Part model, mm, in its own coordinate system. Give positions to 0.01 mm unless a question says otherwise; leave off trailing zeros. Order: outer loops, then holes, each group sorted by start corner. A loop starts at its lowest first (then second) coordinate and runs counter-clockwise, first axis right, second up. Notation, with made-up numbers: (-24, 26) -> (5, 26) arc R12 ccw to (5, 36) -> close; hole circle Ø9 at (13, -31.5). An arc over 180 degrees is marked (long way). Write item = value, one per line. Start each with the question number.
Item 1: Drill centre lines: line 1 along Y through (x, z) = (-13.5, 0.5); line 2 along X through (y, z) = (5.5, -1.3); line 3 along Y through (x, z) = (-2, 0.4). Where is each one in solid material? Low to high.
Item 2: Pull direction X, two halves, no side cores. Call faces 1 (the face through (2, 0, -4)), 2 (the face through (14.219, -14.943, -1.535)), 3 (the face through (-21.083, 0, -2)), 4 (the face through (24.984, -0.901, -1.535)): +X half, -X half, draft (parallel to the pull), parting line (faces both ways), or undercut.
Item 3: Flat gauge pins, fed straight in: P1, Ø1.5, axis at x = 18.5, z = 0.5, coming from the +Y side; P2, Ø1, axis at x = 12.5, z = -2, coming from the -Y side. Where does each tip first touch, or does it go through?
Item 4: Band-saw the part on C-C on y = 21. Write the cut outline in (x, z).
Item 5: Band-saw the part on B-B on x = 20. Write the cut outline in (y, z).
Item 6: Band-saw the part on A-A on z = -2.45. Write the cut outline in (x, y), plus the area to 3 significant figures.
```python
from build123d import *

# Parameters (mm, degrees)
BOSS_EXTRU_1_DEPTH      = 1
BOSS_EXTRU_1_DEPTH_BACK = 4
ESQUISSE1_R             = 25
ESQUISSE1_R_2           = 1.7
ESQUISSE2_W             = 7.120092975
ESQUISSE2_H             = 26.945103847
ENL_V_MAT_EXTRU_1_DEPTH = 36.707142143


with BuildPart() as part:
    # Esquisse1 → Boss.-Extru.1 (new, two sides: drawn at the far end of the back side and taken through both)
    with BuildSketch(Plane.XY.offset(-BOSS_EXTRU_1_DEPTH_BACK)):
        Circle(ESQUISSE1_R)
        with Locations((-13.435028843, 13.435028843)):
            Circle(ESQUISSE1_R_2, mode=Mode.SUBTRACT)
        with Locations((13.435028843, 13.435028843)):
            Circle(ESQUISSE1_R_2, mode=Mode.SUBTRACT)
        with Locations((13.435028843, -13.435028843)):
            Circle(ESQUISSE1_R_2, mode=Mode.SUBTRACT)
        with Locations((-13.435028843, -13.435028843)):
            Circle(ESQUISSE1_R_2, mode=Mode.SUBTRACT)
    extrude(amount=BOSS_EXTRU_1_DEPTH + BOSS_EXTRU_1_DEPTH_BACK)

    # Esquisse2 → Enlèv. mat.-Extru.1 (cut, through all)
    with BuildSketch(Plane(origin=(0, 0, -4), x_dir=(-1, 0, 0), z_dir=(0, 0, -1))):
        with Locations((24.643215129, 0.03752308)):
            Rectangle(ESQUISSE2_W, ESQUISSE2_H)
    extrude(amount=-ENL_V_MAT_EXTRU_1_DEPTH, mode=Mode.SUBTRACT)


solid = part.part
```
Values found:
q1.line_1 = -21.04 to -15.13, -11.74 to 11.74, 15.13 to 21.04
q1.line_2 = -21.08 to 24.39
q1.line_3 = -24.92 to 24.92
q2.face_1 = draft
q2.face_2 = undercut
q2.face_3 = -X half
q2.face_4 = parting line
q3.P1 = 17.61
q3.P2 = -21.93
q4.outline = (-13.56, -4) -> (13.56, -4) -> (13.56, 1) -> (-13.56, 1) -> close
q5.outline = (-15, -4) -> (15, -4) -> (15, 1) -> (-15, 1) -> close
q6.outline = (-21.08, -13.44) arc R25 ccw (long way) to (-21.08, 13.44) -> close; hole circle Ø3.4 at (-13.44, -13.44); hole circle Ø3.4 at (-13.44, 13.44); hole circle Ø3.4 at (13.44, -13.44); hole circle Ø3.4 at (13.44, 13.44)
q6.area = 1,860 mm^2
